Read the model definition and answer for the solid it produces. Units are mm, in the model's axes. A direction names the side the tool comes from. Coordinates: 2 decimals unless noted, no trailing zeros. Loops run counter-clockwise (first coordinate to the right, second up) from the corner with the lowest first, then second, coordinate; pieces in that order, holes last. Notation, with made-up numbers: (-14, 62) - (38, 62) arc R26 cw to (38, 86) - close; hole circle Ø11 at (22, -5.5). An arc over 180 degrees is marked (long way). Use one line per item in the form item = value.
from build123d import *

# Parameters (mm, degrees)
BODY1_W                            = 7.9
BODY1_H                            = 4.8
EXTRUDE_1_DEPTH                    = 6
SKETCH_2_W                         = 6.7
SKETCH_2_H                         = 3.6
CUT_EXTRUDE_1_DEPTH                = 4.2
CHAMFER_1_SIZE                     = 0.35
SKETCH_4_W                         = 0.96
SKETCH_4_H                         = 3.91
CUT_EXTRUDE_3_DEPTH                = 0.45
SKETCH_5_W                         = 0.7
SKETCH_5_H                         = 3.45
CUT_EXTRUDE_4_DEPTH                = 0.4
CUT_EXTRUDE_6_REACH                = 13.02
SKETCH_8_W                         = 2.3
SKETCH_8_H                         = 4.05
CUT_EXTRUDE_7_REACH                = 13.02
SKETCH_15_W                        = 6.7
SKETCH_15_H                        = 1.95
CUT_EXTRUDE_9_DEPTH                = 0.65
CHAMFER_7_SIZE                     = 0.65
SKETCH_10_W                        = 0.5
SKETCH_10_H                        = 2.25
EXTRUDE_2_DEPTH                    = 0.3
CHAMFER_2_SIZE                     = 0.25
PATTERN_LINEAR_3_COUNT             = 2
PATTERN_LINEAR_3_PITCH             = 2
CHAMFER_2_OF_PATTERN_LINEAR_3_SIZE = 0.25
EXTRUDE_5_DEPTH                    = 0.95
SWEEP_START                        = 1.7
SWEEP_1_DEPTH                      = 0.5
CHAMFER_8_SIZE                     = 0.1
PATTERN_LINEAR_5_COUNT             = 3
PATTERN_LINEAR_5_PITCH             = 2
CHAMFER_8_OF_PATTERN_LINEAR_5_SIZE = 0.1
SKETCH_18_R                        = 0.05
CUT_EXTRUDE_10_DEPTH               = 3.4


# Read off the part's stored shape, not the designer's step: По траектории1
with BuildPart() as part:
    # Body1 → Бобышка-Вытянуть1 (new body)
    with BuildSketch(Plane(origin=(0, 0, 0), x_dir=(1, 0, 0), z_dir=(0, 1, 0))):
        with Locations((3.95, -2.4)):
            Rectangle(BODY1_W, BODY1_H)
    extrude(amount=EXTRUDE_1_DEPTH)

    # Эскиз2 → Вырез-Вытянуть1 (cut)
    with BuildSketch(Plane(origin=(0, 6, 0), x_dir=(1, 0, 0), z_dir=(0, 1, 0))):
        with Locations((3.95, -2.55)):
            Rectangle(SKETCH_2_W, SKETCH_2_H)
    extrude(amount=-CUT_EXTRUDE_1_DEPTH, mode=Mode.SUBTRACT)

    # Фаска1
    chamfer_1_edges = [part.edges().sort_by_distance(p)[0] for p in [
        (7.3, 6, 2.55),
        (3.95, 6, 0.75),
        (0.6, 6, 2.55),
        (3.95, 6, 4.35),
    ]]
    chamfer(chamfer_1_edges, length=CHAMFER_1_SIZE)

    # Эскиз4 → Вырез-Вытянуть3 (cut)
    with BuildSketch(Plane.XY.offset(4.8)):
        with Locations((1.25, 1.955)):
            Rectangle(SKETCH_4_W, SKETCH_4_H)
        with Locations((6.65, 1.955)):
            Rectangle(SKETCH_4_W, SKETCH_4_H)
    extrude(amount=-CUT_EXTRUDE_3_DEPTH, mode=Mode.SUBTRACT)

    # Эскиз5 → Вырез-Вытянуть4 (cut)
    with BuildSketch(Plane(origin=(0, 0, 4.8), x_dir=(1, 0, 0), z_dir=(0, 1, 0))):
        with Locations((1.95, 3.075)):
            Rectangle(SKETCH_5_W, SKETCH_5_H)
    cut_extrude_4 = extrude(amount=CUT_EXTRUDE_4_DEPTH, mode=Mode.SUBTRACT)

    # Эскиз8 → Вырез-Вытянуть6 (cut, up to next)
    with BuildSketch(Plane.XY.offset(4.8), mode=Mode.PRIVATE) as cut_extrude_6_sk1:
        with Locations((3.95, 3.975)):
            Rectangle(SKETCH_8_W, SKETCH_8_H)
    cut_extrude_6_tool1 = extrude(cut_extrude_6_sk1.sketch, amount=-CUT_EXTRUDE_6_REACH, mode=Mode.PRIVATE) & part.part
    add(cut_extrude_6_tool1.solids().sort_by_distance((3.95, 3.975, 4.8))[0], mode=Mode.SUBTRACT)

    # Эскиз9 → Вырез-Вытянуть7 (cut, up to next)
    with BuildSketch(Plane.ZY, mode=Mode.PRIVATE) as cut_extrude_7_sk1:
        with BuildLine():
            Line((2.42, 6), (3.42, 6))
            Line((3.42, 6), (3.42, 4.5))
            ThreePointArc((3.42, 4.5), (2.92, 4), (2.42, 4.5))
            Line((2.42, 4.5), (2.42, 6))
        make_face()
    cut_extrude_7_tool1 = extrude(cut_extrude_7_sk1.sketch, amount=-CUT_EXTRUDE_7_REACH, mode=Mode.PRIVATE) & part.part
    cut_extrude_7 = cut_extrude_7_tool1.solids().sort_by_distance((0, 5.05036, 2.92))[0]
    add(cut_extrude_7, mode=Mode.SUBTRACT)

    # Зеркальное отражение1: Вырез-Вытянуть7 across plane
    add(cut_extrude_7.mirror(Plane(origin=(3.95, 0, 0), x_dir=(0, 0, 1), z_dir=(1, 0, 0))), mode=Mode.SUBTRACT)

    # Эскиз15 → Вырез-Вытянуть9 (cut)
    with BuildSketch(Plane(origin=(0, 1.8, 0), x_dir=(1, 0, 0), z_dir=(0, 1, 0))):
        with Locations((3.95, -1.725)):
            Rectangle(SKETCH_15_W, SKETCH_15_H)
    extrude(amount=-CUT_EXTRUDE_9_DEPTH, mode=Mode.SUBTRACT)

    # Фаска7
    chamfer_7_edges = [part.edges().sort_by_distance(p)[0] for p in [
        (3.95, 1.15, 2.7),
    ]]
    chamfer(chamfer_7_edges, length=CHAMFER_7_SIZE - 0.0001)  # a hair under: the kernel refuses the full size

    # Эскиз10 → Бобышка-Вытянуть2 (add)
    with BuildSketch(Plane.XY.offset(0.75)):
        with Locations((2.95, 2.275)):
            Rectangle(SKETCH_10_W, SKETCH_10_H)
    extrude_2 = extrude(amount=EXTRUDE_2_DEPTH)

    # Фаска2
    chamfer_2_edges = [part.edges().sort_by_distance(p)[0] for p in [
        (2.95, 3.4, 1.05),
    ]]
    chamfer(chamfer_2_edges, length=CHAMFER_2_SIZE)

    # Линейный массив3: Бобышка-Вытянуть2 ×2
    with Locations(*[(i * PATTERN_LINEAR_3_PITCH, 0, 0) for i in range(1, PATTERN_LINEAR_3_COUNT)]):
        add(extrude_2)

    # Фаска2 of Линейный массив3
    chamfer_2_of_pattern_linear_3_edges = [part.edges().sort_by_distance(p)[0] for p in [
        (4.95, 3.4, 1.05),
    ]]
    chamfer(chamfer_2_of_pattern_linear_3_edges, length=CHAMFER_2_OF_PATTERN_LINEAR_3_SIZE)

    # Эскиз17 → Бобышка-Вытянуть5 (add)
    with BuildSketch(Plane.ZY):
        Polygon((0, -1.6), (1.95, -1.6), (3.85, 0), (0, 0), align=None)
    extrude_5 = extrude(amount=-EXTRUDE_5_DEPTH)

    # Зеркальное отражение3: Бобышка-Вытянуть5 across plane
    add(extrude_5.mirror(Plane(origin=(3.95, 0, 0), x_dir=(0, 0, 1), z_dir=(1, 0, 0))))

    # По траектории1 outline → По траектории1 (add)
    with BuildSketch(Plane.YZ.offset(SWEEP_START)):
        with BuildLine():
            add(Edge.make_bspline(
                [(-0.5, 2.45), (-0.5, 2.683362296), (-0.405057001, 2.917735205), (-0.152065654, 3.170726552), (-0.050887811, 3.237723146), (0.166472235, 3.327081743), (0.298557942, 3.349954697), (0.4, 3.35)],
                knots=[0.50998091, 0.50998091, 0.50998091, 0.50998091, 0.55448514, 0.55448514, 0.576737255, 0.576737255, 0.59898937, 0.59898937, 0.59898937, 0.59898937], degree=3))
            Line((-0.5, 2.45), (-0.5, -3.4))
            Line((-0.5, -3.4), (0, -3.4))
            Line((0, -3.4), (0, 2.45))
            add(Edge.make_bspline(
                [(0, 2.45), (0, 2.553716576), (0.042196888, 2.657882313), (0.154637487, 2.770322912), (0.199605417, 2.800099176), (0.296209882, 2.839814108), (0.331279974, 2.849979865), (0.4, 2.85)],
                knots=[0.50998091, 0.50998091, 0.50998091, 0.50998091, 0.55448514, 0.55448514, 0.576737255, 0.576737255, 0.59898937, 0.59898937, 0.59898937, 0.59898937], degree=3))
            Line((0.4, 2.85), (0.4, 3.35))
        make_face()
        with BuildLine():
            Line((1.8, 3.35), (1.8, 2.85))
            add(Edge.make_bspline(
                [(1.8, 2.85), (2.1, 2.85), (2.4, 2.85), (3.466666667, 2.85), (4.233333333, 2.85), (5, 2.85)],
                knots=[0.721036083, 0.721036083, 0.721036083, 0.721036083, 0.799494685, 0.799494685, 1, 1, 1, 1], degree=3))
            Line((5, 2.85), (5, 3.35))
            add(Edge.make_bspline(
                [(1.8, 3.35), (2.1, 3.35), (2.4, 3.35), (3.466666667, 3.35), (4.233333333, 3.35), (5, 3.35)],
                knots=[0.721036083, 0.721036083, 0.721036083, 0.721036083, 0.799494685, 0.799494685, 1, 1, 1, 1], degree=3))
        make_face()
    sweep_1 = extrude(amount=SWEEP_1_DEPTH)

    # Фаска8
    chamfer_8_edges = [part.edges().sort_by_distance(p)[0] for p in [
        (1.95, 5, 2.85),
        (2.2, 5, 3.1),
        (1.95, 5, 3.35),
        (1.7, 5, 3.1),
        (1.95, -0.5, -3.4),
        (2.2, -0.25, -3.4),
        (1.95, 0, -3.4),
        (1.7, -0.25, -3.4),
    ]]
    chamfer(chamfer_8_edges, length=CHAMFER_8_SIZE)

    # Линейный массив5: Вырез-Вытянуть4, По траектории1 ×3
    with Locations(*[(i * PATTERN_LINEAR_5_PITCH, 0, 0) for i in range(1, PATTERN_LINEAR_5_COUNT)]):
        add(cut_extrude_4, mode=Mode.SUBTRACT)
        add(sweep_1)

    # Фаска8 of Линейный массив5
    chamfer_8_of_pattern_linear_5_edges = [part.edges().sort_by_distance(p)[0] for p in [
        (3.95, 5, 2.85),
        (4.2, 5, 3.1),
        (3.95, 5, 3.35),
        (3.7, 5, 3.1),
        (3.95, -0.5, -3.4),
        (4.2, -0.25, -3.4),
        (3.95, 0, -3.4),
        (3.7, -0.25, -3.4),
        (5.95, 5, 2.85),
        (6.2, 5, 3.1),
        (5.95, 5, 3.35),
        (5.7, 5, 3.1),
        (5.95, -0.5, -3.4),
        (6.2, -0.25, -3.4),
        (5.95, 0, -3.4),
        (5.7, -0.25, -3.4),
    ]]
    chamfer(chamfer_8_of_pattern_linear_5_edges, length=CHAMFER_8_OF_PATTERN_LINEAR_5_SIZE)

    # Эскиз18 → Вырез-Вытянуть10 (cut)
    with BuildSketch(Plane(origin=(0, 0, 0), x_dir=(-1, 0, 0), z_dir=(0, 0, -1))):
        with Locations(Location((-1.95, -0.25, 0), (0, 0, 90))):
            Circle(SKETCH_18_R)
    extrude(amount=CUT_EXTRUDE_10_DEPTH, mode=Mode.SUBTRACT)


solid = part.part
Item 1: Each of these flat-tipped pins is pushed along its axis until it touches: P1, Ø2, axis at x = 3.5, y = 2, coming from the +Z side; P2, Ø3, axis at x = 4.5, y = 4.5, coming from the -Z side. Where does it stop, or does it pass through?
Results below:
P1 = 4.8
P2 = 0
Item 2: For a pull along Z with two mould halves and no side action, classify faces 1 (the flat face through (0.5, -0.8, 2.9)), 2 (the flat face through (6.95, -1, 1)), 3 (the flat face through (4, 3, 0.75)) as +Z half, -Z half, draft (parallel to the pull), parting line (faces both ways), or undercut.
Results below:
face_1 = +Z half
face_2 = draft
face_3 = undercut
Item 3: The part is cut by section A-A on z = -1.75. Give the vertices of the cut face in (x, y), plus the area to 3 significant figures.
Results below:
outline = (1.7, -0.5) - (2.2, -0.5) - (2.2, 0) - (1.7, 0) - close; (3.7, -0.5) - (4.2, -0.5) - (4.2, 0) - (3.7, 0) - close; (5.7, -0.5) - (6.2, -0.5) - (6.2, 0) - (5.7, 0) - close; hole circle Ø0.1 at (1.95, -0.25)
area = 0.742 mm²
Item 4: Which of the six approach directions +Z, -Z, +X, -X, +Y, -Y give full straight-line access (tool end or side, diameter ignored) to faces 4 (the flat face through (0.95, -1, 1)), 5 (the flat face through (5, 0, 3)), 6 (the flat face through (5.4, 4.2, 4.35))?
Results below:
face_4 = +Z, -Z, -Y
face_5 = +Z, -Y
face_6 = +Y
Item 5: Find the intervals of material crossed by L1, parallel to X at y = 3.25, z = 2; L2, parallel to Z at x = 6, y = 3.5; L3, parallel to Z at x = 6.25, y = 4.75, in increasing order.
Results below:
L1 = 0 to 0.6, 7.3 to 7.9
L2 = 0 to 0.75, 2.85 to 3.35, 4.35 to 4.8
L3 = 0 to 0.75, 4.35 to 4.8
Item 6: The part is cut by section C-C on x = 7.5. Give the vertices of the cut face in (y, z), plus the area to 3 significant figures.
Results below:
outline = (-1.6, 0) - (6, 0) - (6, 0.4) - (5.85, 0.55) - (5.85, 2.42) - (4.5, 2.42) arc R0.5 cw to (4.5, 3.42) - (5.85, 3.42) - (5.85, 4.55) - (6, 4.7) - (6, 4.8) - (0, 4.8) - (0, 3.85) - (-1.6, 1.95) - close
area = 31.1 mm²
